from build123d import *

# Parameters (mm, degrees)
F0_R     = 25
F1_DEPTH = 4
F3_DEPTH = 25


with BuildPart() as f1:
    # F0 (on Front) → F1 (new body)
    with BuildSketch(Plane.XZ):
        with Locations((3.8093454119, 0)):
            Circle(F0_R)
    extrude(amount=F1_DEPTH)

    # F2 (on face) → F3 (cut)
    with BuildSketch(Plane.XZ.offset(4)):
        with BuildLine():
            ThreePointArc((-11.7582220598, 19.5614632125), (-13.1639870123, 18.354998949), (-14.4765553037, 17.0477516118))
            Line((-14.4765553037, 17.0477516118), (-14.4765553037, 9.326151153))
            Line((-14.4765553037, 9.326151153), (-11.7582220598, 19.5614632125))
        make_face()
        with BuildLine():
            ThreePointArc((2.7612951022, 24.9780221504), (0.9145785092, 24.8318409422), (-0.9162435852, 24.5493138118))
            Line((-0.9162435852, 24.5493138118), (-5.4669922591, 18.3112211424))
            Line((-5.4669922591, 18.3112211424), (2.7612951022, 24.9780221504))
        make_face()
        with BuildLine():
            ThreePointArc((17.6835243201, 20.7968064765), (16.1054546899, 21.7670782749), (14.4598699542, 22.6178320573))
            Line((14.4598699542, 22.6178320573), (7.106992246, 20.2602266935))
            Line((7.106992246, 20.2602266935), (17.6835243201, 20.7968064765))
        make_face()
        with BuildLine():
            ThreePointArc((27.2746171782, 8.6244432247), (26.5715658455, 10.338342272), (25.7435324005, 11.9954758618))
            Line((25.7435324005, 11.9954758618), (18.4138599684, 14.4242647952))
            Line((18.4138599684, 14.4242647952), (27.2746171782, 8.6244432247))
        make_face()
        with BuildLine():
            ThreePointArc((27.8492079184, -6.8618518398), (28.2913215022, -5.0628891666), (28.5990101913, -3.2361273346))
            Line((28.5990101913, -3.2361273346), (24.1089607469, 3.0457967044))
            Line((24.1089607469, 3.0457967044), (27.8492079184, -6.8618518398))
        make_face()
        with BuildLine():
            Line((22.0039590385, -9.5030150632), (19.1865107481, -19.7114886861))
            ThreePointArc((19.1865107481, -19.7114886861), (20.603907642, -18.5187116048), (21.9290894609, -17.2242525411))
            Line((21.9290894609, -17.2242525411), (22.0039590385, -9.5030150632))
        make_face()
        with BuildLine():
            Line((12.9076991878, -18.4003048584), (4.6151565122, -24.9870099946))
            ThreePointArc((4.6151565122, -24.9870099946), (6.4632036846, -24.8587416469), (8.2966791322, -24.5939796715))
            Line((8.2966791322, -24.5939796715), (12.9076991878, -18.4003048584))
        make_face()
        with BuildLine():
            Line((0.3154079719, -20.2272999058), (-10.2658296583, -20.661303123))
            ThreePointArc((-10.2658296583, -20.661303123), (-8.6972420842, -21.6468304655), (-7.0599837172, -22.5135000452))
            Line((-7.0599837172, -22.5135000452), (0.3154079719, -20.2272999058))
        make_face()
        with BuildLine():
            Line((-10.934342035, -14.2819795819), (-19.7384469382, -8.3965156722))
            ThreePointArc((-19.7384469382, -8.3965156722), (-19.0520468287, -10.1171510229), (-18.2401200772, -11.7822354264))
            Line((-18.2401200772, -11.7822354264), (-10.934342035, -14.2819795819))
        make_face()
        with BuildLine():
            Line((-16.5188480842, -2.8488259856), (-20.1628536664, 7.0946227067))
            ThreePointArc((-20.1628536664, 7.0946227067), (-20.6223894281, 5.3000313871), (-20.9477761583, 3.4763388154))
            Line((-20.9477761583, 3.4763388154), (-16.5188480842, -2.8488259856))
        make_face()
    extrude(amount=-F3_DEPTH, mode=Mode.SUBTRACT)


solid = f1.part
Could you check a few things on this model? Use its own coordinates, in mm. Give positions to 0.01 mm unless a question says otherwise; leave off trailing zeros. Order: outer loops, then holes, each group sorted by start corner. A loop starts at its lowest first (then second) coordinate and runs counter-clockwise, first axis right, second up. Notation, with made-up numbers: (42, 24) -> (84, 24) arc R16 cw to (84, 46) -> close; hole circle Ø7 at (-19.75, -17.5). An arc over 180 degrees is marked (long way). Answer in a Markdown table with one row per item. Add a question column.
Item 1: Please list where these lines run through material, in increasing order: probe 1 along X at (y, z) = (-1.05, 2); probe 2 along X at (y, z) = (-1.35, 0); probe 3 along Z at (x, y) = (-2, -0.15).
Item 2: Imagine slicing it at A-A (x = -3). List the corners of the cut face in (y, z) for me (3 decimals), and give its area (3 significant figures).
Item 3: Imagine slicing it at B-B (z = -13.5). List the corners of the cut face in (x, y) for me.
Item 4: I'm going to push flat-ended pins straight in: P1, Ø8, axis at x = 19.5, z = -2, coming from the +Y side; P2, Ø2, axis at x = 2.5, y = -3, coming from the +Z side. Where does each tip first touch, or does it pass through?
Item 5: Imagine slicing it at D-D (x = 15.5). List the corners of the cut face in (y, z) for me, and give its area (3 significant figures).
Item 6: We'd pull the mould along X, two halves only. Please class faces 1 (the flat face through (12.321, -2.028, 20.525)), 2 (the cylindrical face through (28.664, -1.972, 2.69)), 3 (the cylindrical face through (-14.85, -1.97, -16.64)): pulls with the +X half, pulls with the -X half, needs draft (parallel to the pull), parting line crosses it, or undercut.
Result:
| question | item | result |
|---|---|---|
| 1 | probe 1 | -21.11 to -19.91, -18.3 to 24.5, 24.86 to 28.73 |
| 1 | probe 2 | -21.19 to -18.51, -17.56 to 25.26, 26.29 to 28.81 |
| 1 | probe 3 | -24.32 to -20.95, -20.32 to 21.12, 23.06 to 24.32 |
| 2 | outline | (-4, -24.055) -> (0, -24.055) -> (0, -21.255) -> (-4, -21.255) -> close; (-4, -20.363) -> (0, -20.363) -> (0, 20.31) -> (-4, 20.31) -> close; (-4, 21.693) -> (0, 21.693) -> (0, 24.055) -> (-4, 24.055) -> close |
| 2 | area | 183 mm2 |
| 3 | outline | (-17.23, -4) -> (-13.22, -4) -> (-13.22, 0) -> (-17.23, 0) -> close; (-12.1, -4) -> (20.9, -4) -> (20.9, 0) -> (-12.1, 0) -> close; (21.97, -4) -> (24.85, -4) -> (24.85, 0) -> (21.97, 0) -> close |
| 4 | P1 | y = 0 |
| 4 | P2 | z = 25 |
| 5 | outline | (-4, -22.1) -> (0, -22.1) -> (0, 20.69) -> (-4, 20.69) -> close |
| 5 | area | 171 mm2 |
| 6 | face 1 | undercut |
| 6 | face 2 | pulls with the +X half |
| 6 | face 3 | pulls with the -X half |
